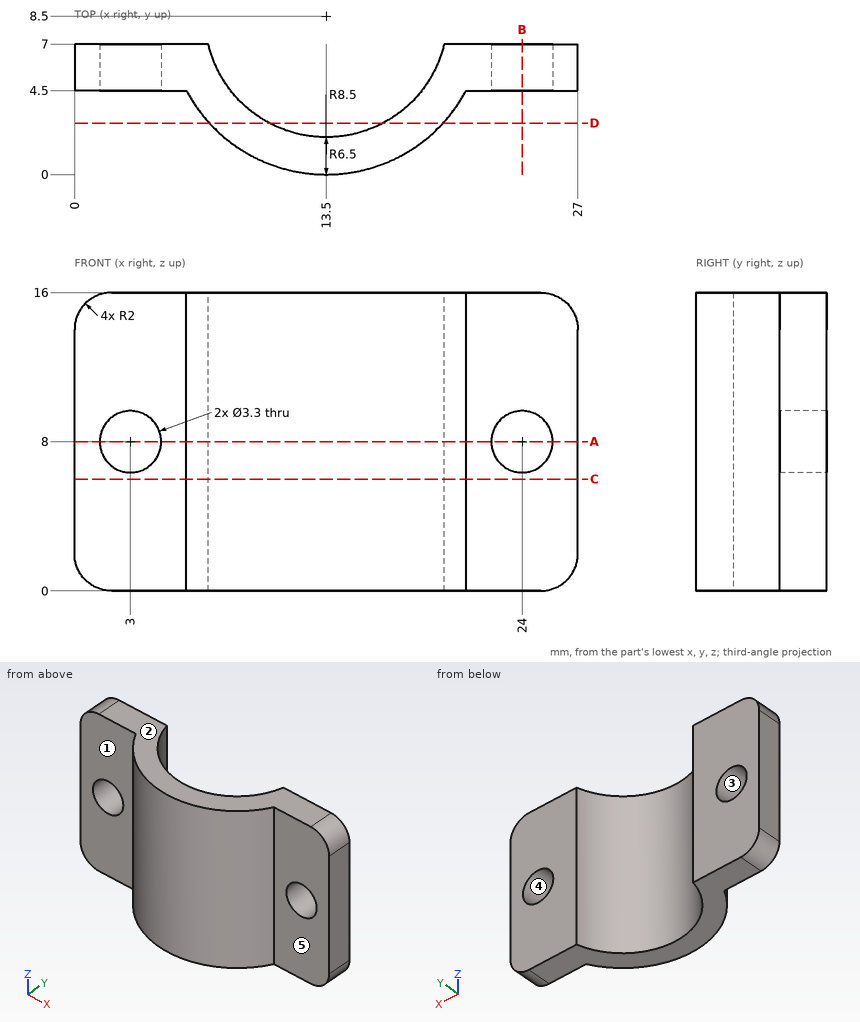
The figure shows three views and two pictorial views of one solid part (mm, origin at its lowest corner). Answer the questions. A direction names the side the tool comes from. Give positions to 0.01 mm unless a question says otherwise; leave off trailing zeros. Write each loop counter-clockwise with the first axis right and the second up, starting at its lowest first coordinate (ties: lowest second). Pieces come first, ordered by that corner, then holes.
Q1. The part is cut by section A-A on z = 8. Give the vertices of the cut face in (x, y).
Answer:
outline: (0, 4.5) - (1.35, 4.5) - (1.35, 7) - (0, 7) - close; (4.65, 4.5) - (6, 4.5) arc R8.5 ccw to (21, 4.5) - (22.35, 4.5) - (22.35, 7) - (19.82, 7) arc R6.5 cw to (7.18, 7) - (4.65, 7) - close; (25.65, 4.5) - (27, 4.5) - (27, 7) - (25.65, 7) - close
Q2. The part is cut by section C-C on z = 6. Give the vertices of the cut face in (x, y), and give its area (4 significant figures).
Answer:
outline: (0, 4.5) - (6, 4.5) arc R8.5 ccw to (21, 4.5) - (27, 4.5) - (27, 7) - (19.82, 7) arc R6.5 cw to (7.18, 7) - (0, 7) - close
area: 68.55 mm2
Q3. A tool of negligible diameter and unlimited length cuts with its end or side. For the marked faces 4 and 5, from which of +Z, -Z, +X, -X, +Y, -Y can it reach the whole face along a straight path? Write none if from no direction.
Answer:
face 4: +Y, -Y
face 5: +Z, -Z, +X, -Y
Q4. Straight lines are drawn through the part: L1, parallel to X at y = 6, z = 8; L2, parallel to Y at x = 23.25, z = 3.75; L3, parallel to X at y = 6.55, z = 8. For each, find the intervals that lie inside material, in ascending order.
Answer:
L1: x = 0 to 1.35, 4.65 to 7.5, 19.5 to 22.35, 25.65 to 27
L2: y = 4.5 to 7
L3: x = 0 to 1.35, 4.65 to 7.3, 19.7 to 22.35, 25.65 to 27
Q5. The part is cut by section D-D on y = 2.75. Give the vertices of the cut face in (x, z).
Answer:
outline: (7.24, 0) - (10.47, 0) - (10.47, 16) - (7.24, 16) - close; (16.53, 0) - (19.76, 0) - (19.76, 16) - (16.53, 16) - close
Q6. The part is cut by section B-B on x = 24. Give the vertices of the cut face in (y, z).
Answer:
outline: (4.5, 0) - (7, 0) - (7, 6.35) - (4.5, 6.35) - close; (4.5, 9.65) - (7, 9.65) - (7, 16) - (4.5, 16) - close
Q7. Given pin 1 (3 mm diameter, centred on x = 9, z = 14, fed in from -Y); pin 2 (5 mm diameter, centred on x = 24.5, z = 5.5, fed in from -Y), each flat-ended and moving along its own axis, determine where each tip first touches the part or whether it passes through.
Answer:
pin 1: stops at y = 0.55
pin 2: stops at y = 4.5
Q8. For a pull along Z with two mould halves and no side action, classify the marked faces 1, 2 and 3 as released by +Z, released by -Z, zero draft, split by the parting line, or undercut.
Answer:
face 1: zero draft
face 2: released by +Z
face 3: undercut
